For this review, take the finished solid that the model builds, in its own axes (mm). A direction names the side the tool comes from. Coordinates: 2 decimals unless noted, no trailing zeros. Write each loop counter-clockwise with the first axis right and the second up, starting at its lowest first coordinate (ties: lowest second). Pieces come first, ordered by that corner, then holes.
1) We need section D-D on x = 105.5. Write out the cut boundary in (y, z), then the cut area to 3 significant figures.
2) We need section C-C on y = -10. Give the number of separate pieces and of enclosed holes in the cut face, then the cut area to 3 significant figures.
3) We need section A-A on z = -32.5. Write out the cut boundary in (x, y).
4) Mouldability with a two-part tool opening along Z and no side actions: class faces 1 (the face through (69.635, -19.119, 46.391)), 2 (the face through (68.21, -12.32, -33.26)), 3 (the face through (69.116, -24.034, 30.424)), 4 (the face through (-49.983, -12.325, 1.285)) as pulls with the +Z half, pulls with the -Z half, needs draft (parallel to the pull), parting line crosses it, or undercut.
5) To check wall thickness, follow line 1 along Z through (x, y) = (0, -19.5); line 2 along Z through (x, y) = (120, -18.5); line 3 along X through (y, z) = (-21.5, -2). State the ranges of each line that lie inside material, in increasing order.
6) We need section B-B on x = -0.5. Write out the cut boundary in (y, z).
7) Insertion check: P1, Ø1, axis at x = 95, z = -18.5, coming from the +Y side; P2, Ø12, axis at y = -16.5, z = 37.5, coming from the -X side; P3, Ø2, axis at x = -16.5, y = -12.5, coming from the -Z side; P4, Ø12, axis at y = -8.5, z = -16.5, coming from the +X side. Each pin has a flat end and moves straight along its axis. Give the tip position at first contact, or say it passes through.
8) For faces 5 (the face through (-29, -25, -28)), 6 (the face through (-47.484, -13.592, 1.221)), 7 (the face through (73.9, -12.4, 57)), list the 3-axis set-ups (+Z, -Z, +X, -X, +Y, -Y) from which the entire face can be reached by the end or side of a thin tool; tool diameter is ignored.
from build123d import *

# Parameters (mm, degrees)
F0_R     = 40
F1_DEPTH = 25
F2_R     = 9.27978
F3_DEPTH = 26.9
F4_R     = 2
F5_R     = 4.5
F6_DEPTH = 25.001
F7_T     = -2.5


with BuildPart() as f1:
    # F0 (on Front) → F1 (new body)
    with BuildSketch(Plane.XZ):
        with BuildLine():
            ThreePointArc((13.125, -48.2466), (39.725621, -30.362395), (50, 0))
            ThreePointArc((50, 0), (39.725621, 30.362395), (13.125, 48.2466))
            ThreePointArc((13.125, 48.2466), (-50, 0), (13.125, -48.2466))
        make_face()
        Circle(F0_R, mode=Mode.SUBTRACT)
        with BuildLine():
            ThreePointArc((13.125, 48.2466), (39.725621, 30.362395), (50, 0))
            ThreePointArc((50, 0), (39.725621, -30.362395), (13.125, -48.2466))
            Line((13.125, -48.2466), (124.85625, -17.851242))
            ThreePointArc((124.85625, -17.851242), (101.5, 0), (124.85625, 17.851242))
            Line((124.85625, 17.851242), (13.125, 48.2466))
        make_face()
        with BuildLine():
            ThreePointArc((138.5, 0), (134.69848, 11.234086), (124.85625, 17.851242))
            ThreePointArc((124.85625, 17.851242), (101.5, 0), (124.85625, -17.851242))
            ThreePointArc((124.85625, -17.851242), (134.69848, -11.234086), (138.5, 0))
        make_face()
    extrude(amount=F1_DEPTH)

    # F2 (on face) → F3 (join)
    with BuildSketch(Plane(origin=(13.125, 0, 48.2466), x_dir=(0.964932, 0, -0.2625), z_dir=(0.2625, 0, 0.964932))):
        with Locations((56.484982, -12.5)):
            Circle(F2_R)
    extrude(amount=F3_DEPTH)

    # F4
    f4_edges = [f1.edges().sort_by_distance(p)[0] for p in [
        (65.73606, -12.5, 61.811904),
        (58.67481, -12.5, 35.855234),
    ]]
    fillet(f4_edges, radius=F4_R)

    # F5 (on face) → F6 (cut, through all)
    with BuildSketch(Plane.XZ.offset(25)):
        with Locations((120, 0)):
            Circle(F5_R)
    extrude(amount=-F6_DEPTH, mode=Mode.SUBTRACT)

    # F7
    f7_openings = [f1.faces().sort_by_distance(p)[0] for p in [
        (52.131114, -25, 0),
    ]]
    offset(amount=F7_T, openings=f7_openings)


solid = f1.part
Result:
1. outline: (-25, -23.12) - (0, -23.12) - (0, 23.12) - (-25, 23.12) - (-25, 20.53) - (-2.5, 20.53) - (-2.5, -20.53) - (-25, -20.53) - close
1. area: 232 mm2
2. separate pieces: 3
2. enclosed holes: 3
2. area: 2,010 mm2
3. outline: (-38, -25) - (-34.64, -25) - (-34.64, -2.5) - (-27.39, -2.5) - (-27.39, -25) - (-23.32, -25) - (-23.32, 0) - (-38, 0) - close; (23.32, -25) - (27.39, -25) - (27.39, -2.5) - (61.48, -2.5) - (61.48, -25) - (71.01, -25) - (71.01, 0) - (23.32, 0) - close
4. face 1: undercut
4. face 2: pulls with the -Z half
4. face 3: undercut
4. face 4: parting line crosses it
5. line 1: z = -50 to -47.5, -42.5 to -40, 40 to 42.5, 47.5 to 50
5. line 2: z = -19.17 to -16.58, -7 to -4.5, 4.5 to 7, 16.58 to 19.17
5. line 3: x = -49.96 to -47.46, -42.45 to -39.95, 39.95 to 42.45, 113.29 to 115.97, 124.03 to 126.71, 135.87 to 138.39
6. outline: (-25, -50) - (0, -50) - (0, -40) - (-25, -40) - (-25, -42.5) - (-2.5, -42.5) - (-2.5, -47.5) - (-25, -47.5) - close; (-25, 40) - (0, 40) - (0, 50) - (-25, 50) - (-25, 47.5) - (-2.5, 47.5) - (-2.5, 42.5) - (-25, 42.5) - close
7. P1: stops at y = 0
7. P2: stops at x = -38.83
7. P3: stops at z = -47.54
7. P4: stops at x = 135.23
8. face 5: +Z, -Z, +X, -X, -Y
8. face 6: -Y
8. face 7: none
